from build123d import *

# Parameters (mm, degrees)
SKETCH1_W          = 31.75
SKETCH1_H          = 38.1
EXTRUDE1_DEPTH     = 6.35
FILLET1_R          = 12.7
SKETCH2_R          = 2.032
CUT_EXTRUDE1_DEPTH = 12.7


with BuildPart() as part:
    # Sketch1 → Extrude1 (new, symmetric)
    with BuildSketch(Plane.XY):
        with Locations((22.225, 54.61)):
            Rectangle(SKETCH1_W, SKETCH1_H)
    extrude(amount=EXTRUDE1_DEPTH, both=True)

    # Fillet1
    fillet1_edges = [part.edges().sort_by_distance(p)[0] for p in [
        (38.1, 35.56, 0),
        (6.35, 35.56, 0),
    ]]
    fillet(fillet1_edges, radius=FILLET1_R)

    # Sketch2 → Cut-Extrude1 (cut)
    with BuildSketch(Plane(origin=(0, 73.66, 0), x_dir=(-1, 0, 0), z_dir=(0, 1, 0))):
        with Locations(Location((-22.225, 0, 0), (0, 0, 90))):
            Circle(SKETCH2_R)
    extrude(amount=-CUT_EXTRUDE1_DEPTH, mode=Mode.SUBTRACT)


solid = part.part
Build history of the part. All positions in model axes, mm. A direction names the side the tool comes from. Give positions to 0.01 mm unless a question says otherwise; leave off trailing zeros. Order: outer loops, then holes, each group sorted by start corner. A loop starts at its lowest first (then second) coordinate and runs counter-clockwise, first axis right, second up. Notation, with made-up numbers: M -0.5,-19 L 27.5,-19 A23 ccw 27.5,-10 Z; hole C -4.5,-8.75 d9. An arc over 180 degrees is marked long. Put each result on its own line as item: value.
Item 1: Cut at A-A on z = 0. Write the cut outline in (x, y), then the cut area to 3 significant figures.
Results are:
outline: M 6.35,48.26 A12.7 ccw 19.05,35.56 L 25.4,35.56 A12.7 ccw 38.1,48.26 L 38.1,73.66 L 24.26,73.66 L 24.26,60.96 L 20.19,60.96 L 20.19,73.66 L 6.35,73.66 Z
area: 1,090 mm2
Item 2: Cut at D-D on z = 5. Write the cut outline in (x, y), then the cut area to 3 significant figures.
Results are:
outline: M 6.35,48.26 A12.7 ccw 19.05,35.56 L 25.4,35.56 A12.7 ccw 38.1,48.26 L 38.1,73.66 L 6.35,73.66 Z
area: 1,140 mm2
Item 3: Drop flat-ended pins along their axis: pin 1 Ø5 at (y, z) = (41, 3.5) entering from -X; pin 2 Ø2.5 at (x, z) = (22.225, 0) entering from +Y. Give the stop position or say it passes through.
Results are:
pin 1: x = 7.28
pin 2: y = 60.96
Item 4: Pull direction X, two halves, no side cores. Call faces 1 (the face through (20.24, 67.4, -0.44)), 2 (the face through (22, 55, -6.35)), 3 (the face through (6.35, 61, 0)): +X half, -X half, draft (parallel to the pull), parting line (faces both ways), or undercut.
Results are:
face 1: undercut
face 2: draft
face 3: -X half
Item 5: Cut at C-C on x = 33. Write the cut outline in (y, z).
Results are:
outline: M 38.09,-6.35 L 73.66,-6.35 L 73.66,6.35 L 38.09,6.35 Z
Item 6: Wall check: probe 1 along X at (y, z) = (69.5, 0); probe 2 along Z at (x, y) = (22, 67); probe 3 along Z at (x, y) = (21, 70.5). Give the ranges that are in metal, low to high.
Results are:
probe 1: 6.35 to 20.19, 24.26 to 38.1
probe 2: -6.35 to -2.02, 2.02 to 6.35
probe 3: -6.35 to -1.62, 1.62 to 6.35
Item 7: Cut at B-B on y = 67. Write the cut outline in (x, z) (3 decimals).
Results are:
outline: M 6.35,-6.35 L 38.1,-6.35 L 38.1,6.35 L 6.35,6.35 Z; hole C 22.225,0 d4.064
Item 8: Which spindle directions (+Z, -Z, +X, -X, +Y, -Y) get a long thin tool onto all of the face, cutting with end or side? Do faces 4 (the face through (22, 60.96, 0)), 5 (the face through (22, 35.56, 0)). Say none if no direction does.
Results are:
face 4: +Y
face 5: +Z, -Z, +X, -X, -Y
